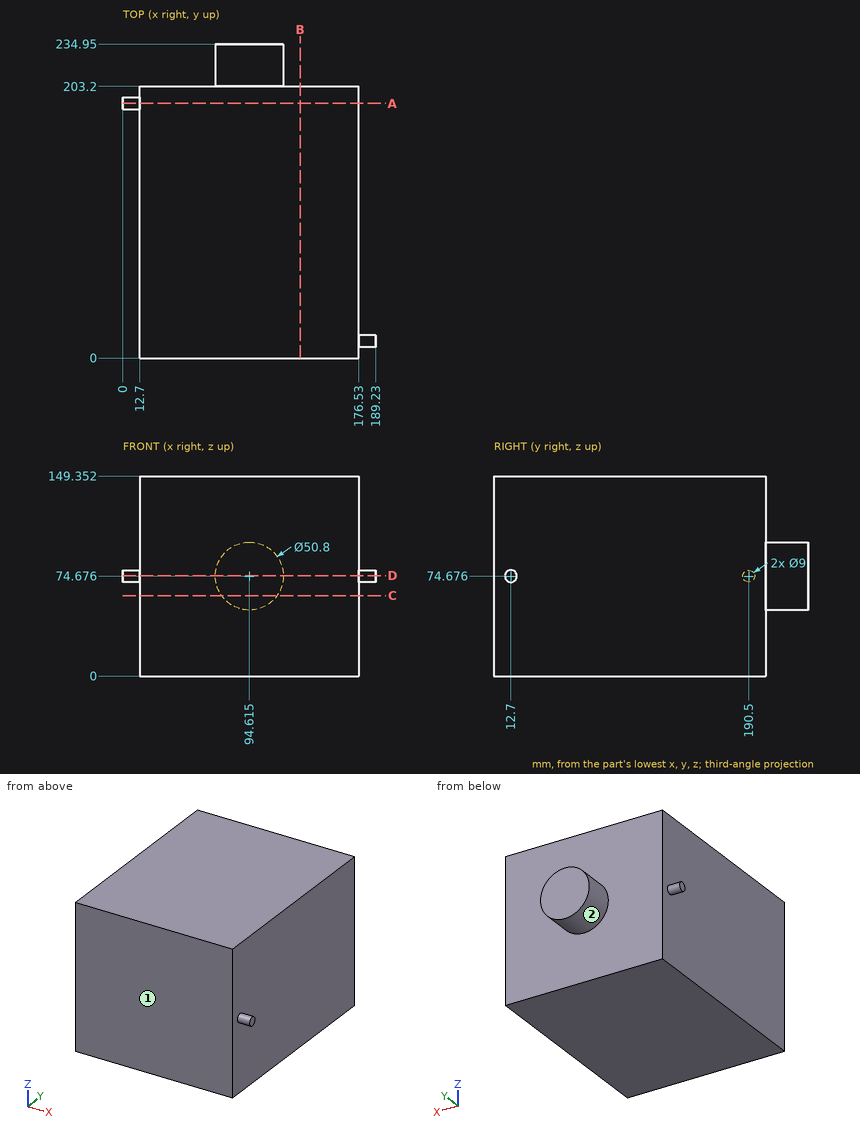
The figure shows three views and two pictorial views of one solid part (mm, origin at its lowest corner). Answer the questions. A direction names the side the tool comes from. Coordinates: 2 decimals unless noted, no trailing zeros. Write each loop counter-clockwise with the first axis right and the second up, starting at its lowest first coordinate (ties: lowest second). Pieces come first, ordered by that corner, then holes. Notation, with made-up numbers: (0.25, 18) -> (52.25, 18) arc R22 ccw to (52.25, 55) -> close; hole circle Ø7 at (-27, 23). An arc over 180 degrees is marked (long way). Return JSON: item names as keys, results as strings.
(1) The part is cut by section A-A on y = 190.5. Give the vertices of the cut face in (x, z), then the cut area to 3 significant figures.
Answers below:
{"outline": "(0, 70.18) -> (12.7, 70.18) -> (12.7, 0) -> (176.53, 0) -> (176.53, 149.35) -> (12.7, 149.35) -> (12.7, 79.18) -> (0, 79.18) -> close", "area": "24,600 mm^2"}
(2) Each of these flat-tipped pins is pushed along its axis until it touches: P1, Ø10, axis at x = 102.5, z = 27.5, coming from the -Y side; P2, Ø5, axis at x = 113.5, z = 120, coming from the +Y side; P3, Ø6, axis at y = 77, z = 44, coming from the -X side; P4, Ø6, axis at y = 79.5, z = 128, coming from the +X side. Where does it stop, or does it pass through?
Answers below:
{"P1": "y = 0", "P2": "y = 203.2", "P3": "x = 12.7", "P4": "x = 176.53"}
(3) Consider line 1 along X through (y, z) = (73.5, 74); line 2 along Y through (x, z) = (145, 143); line 3 along Z through (x, y) = (83, 225.5). Determine where each line is inside the solid, lowest interval first. Write a range as from..to.
Answers below:
{"line 1": "12.7..176.53", "line 2": "0..203.2", "line 3": "52.09..97.26"}
(4) Which of the six approach directions +Z, -Z, +X, -X, +Y, -Y give full straight-line access (tool end or side, diameter ignored) to the marked faces 1 and 2?
Answers below:
{"face 1": "+Z, -Z, +X, -X, -Y", "face 2": "+Y"}
(5) The part is cut by section C-C on z = 60. Give the vertices of the cut face in (x, y).
Answers below:
{"outline": "(12.7, 0) -> (176.53, 0) -> (176.53, 203.2) -> (115.35, 203.2) -> (115.35, 234.95) -> (73.88, 234.95) -> (73.88, 203.2) -> (12.7, 203.2) -> close"}
(6) The part is cut by section D-D on z = 75. Give the vertices of the cut face in (x, y).
Answers below:
{"outline": "(0, 186.01) -> (12.7, 186.01) -> (12.7, 0) -> (176.53, 0) -> (176.53, 8.21) -> (189.23, 8.21) -> (189.23, 17.19) -> (176.53, 17.19) -> (176.53, 203.2) -> (120.01, 203.2) -> (120.01, 234.95) -> (69.22, 234.95) -> (69.22, 203.2) -> (12.7, 203.2) -> (12.7, 194.99) -> (0, 194.99) -> close"}
(7) The part is cut by section B-B on x = 132.5. Give the vertices of the cut face in (y, z).
Answers below:
{"outline": "(0, 0) -> (203.2, 0) -> (203.2, 149.35) -> (0, 149.35) -> close"}
